from build123d import *

# Parameters (mm, degrees)
F0_R          = 3
F0_R_2        = 2.5
F1_DEPTH      = 800
F2_R          = 2
F3_R          = 7
F6_DEPTH      = 30
F6_DEPTH_BACK = 30


# Not quite as in the source:
# - a feature names something its author has since deleted; it is built from what else it names


with BuildPart() as f1:
    # F0 (on Top) → F1 (new body)
    with BuildSketch(Plane.XY):
        with BuildLine():
            Line((18.15, -30), (30, -30))
            Line((30, -30), (30, -18.15))
            Line((30, -18.15), (27.5, -18.15))
            Line((27.5, -18.15), (27.5, -20.15))
            Line((27.5, -20.15), (21.5477069044, -20.15))
            ThreePointArc((21.5477069044, -20.15), (19.5, -15), (21.5477069044, -9.85))
            Line((21.5477069044, -9.85), (27.5, -9.85))
            Line((27.5, -9.85), (27.5, -11.85))
            Line((27.5, -11.85), (30, -11.85))
            Line((30, -11.85), (30, 11.85))
            Line((30, 11.85), (27.5, 11.85))
            Line((27.5, 11.85), (27.5, 9.85))
            Line((27.5, 9.85), (21.5477069044, 9.85))
            ThreePointArc((21.5477069044, 9.85), (19.5, 15), (21.5477069044, 20.15))
            Line((21.5477069044, 20.15), (27.5, 20.15))
            Line((27.5, 20.15), (27.5, 18.15))
            Line((27.5, 18.15), (30, 18.15))
            Line((30, 18.15), (30, 30))
            Line((30, 30), (18.15, 30))
            Line((18.15, 30), (18.15, 27.5))
            Line((18.15, 27.5), (20.15, 27.5))
            Line((20.15, 27.5), (20.15, 21.5477069044))
            ThreePointArc((20.15, 21.5477069044), (15, 19.5), (9.85, 21.5477069044))
            Line((9.85, 21.5477069044), (9.85, 27.5))
            Line((9.85, 27.5), (11.85, 27.5))
            Line((11.85, 27.5), (11.85, 30))
            Line((11.85, 30), (-11.85, 30))
            Line((-11.85, 30), (-11.85, 27.5))
            Line((-11.85, 27.5), (-9.85, 27.5))
            Line((-9.85, 27.5), (-9.85, 21.5477069044))
            ThreePointArc((-9.85, 21.5477069044), (-15, 19.5), (-20.15, 21.5477069044))
            Line((-20.15, 21.5477069044), (-20.15, 27.5))
            Line((-20.15, 27.5), (-18.15, 27.5))
            Line((-18.15, 27.5), (-18.15, 30))
            Line((-18.15, 30), (-30, 30))
            Line((-30, 30), (-30, 18.15))
            Line((-30, 18.15), (-27.5, 18.15))
            Line((-27.5, 18.15), (-27.5, 20.15))
            Line((-27.5, 20.15), (-21.5477069044, 20.15))
            ThreePointArc((-21.5477069044, 20.15), (-19.5, 15), (-21.5477069044, 9.85))
            Line((-21.5477069044, 9.85), (-27.5, 9.85))
            Line((-27.5, 9.85), (-27.5, 11.85))
            Line((-27.5, 11.85), (-30, 11.85))
            Line((-30, 11.85), (-30, -11.85))
            Line((-30, -11.85), (-27.5, -11.85))
            Line((-27.5, -11.85), (-27.5, -9.85))
            Line((-27.5, -9.85), (-21.5477069044, -9.85))
            ThreePointArc((-21.5477069044, -9.85), (-19.5, -15), (-21.5477069044, -20.15))
            Line((-21.5477069044, -20.15), (-27.5, -20.15))
            Line((-27.5, -20.15), (-27.5, -18.15))
            Line((-27.5, -18.15), (-30, -18.15))
            Line((-30, -18.15), (-30, -30))
            Line((-30, -30), (-18.15, -30))
            Line((-18.15, -30), (-18.15, -27.5))
            Line((-18.15, -27.5), (-20.15, -27.5))
            Line((-20.15, -27.5), (-20.15, -21.5477069044))
            ThreePointArc((-20.15, -21.5477069044), (-15, -19.5), (-9.85, -21.5477069044))
            Line((-9.85, -21.5477069044), (-9.85, -27.5))
            Line((-9.85, -27.5), (-11.85, -27.5))
            Line((-11.85, -27.5), (-11.85, -30))
            Line((-11.85, -30), (11.85, -30))
            Line((11.85, -30), (11.85, -27.5))
            Line((11.85, -27.5), (9.85, -27.5))
            Line((9.85, -27.5), (9.85, -21.5477069044))
            ThreePointArc((9.85, -21.5477069044), (15, -19.5), (20.15, -21.5477069044))
            Line((20.15, -21.5477069044), (20.15, -27.5))
            Line((20.15, -27.5), (18.15, -27.5))
            Line((18.15, -27.5), (18.15, -30))
        make_face()
        with Locations((-25, -25)):
            Circle(F0_R, mode=Mode.SUBTRACT)
        with Locations((-15, -15)):
            Circle(F0_R_2, mode=Mode.SUBTRACT)
        with Locations((25, -25)):
            Circle(F0_R, mode=Mode.SUBTRACT)
        with Locations((15, -15)):
            Circle(F0_R_2, mode=Mode.SUBTRACT)
        with Locations((-25, 25)):
            Circle(F0_R, mode=Mode.SUBTRACT)
        with Locations((-15, 15)):
            Circle(F0_R_2, mode=Mode.SUBTRACT)
        Polygon((-7, 22), (-7, 27.5), (0, 27.5), (7, 27.5), (7, 22), (10, 16), (10, 10), (16, 10), (22, 7), (27.5, 7), (27.5, 0), (27.5, -7), (22, -7), (16, -10), (10, -10), (10, -16), (7, -22), (7, -27.5), (0, -27.5), (-7, -27.5), (-7, -22), (-10, -16), (-10, -10), (-16, -10), (-22, -7), (-27.5, -7), (-27.5, 0), (-27.5, 7), (-22, 7), (-16, 10), (-10, 10), (-10, 16), align=None, mode=Mode.SUBTRACT)
        with Locations((15, 15)):
            Circle(F0_R_2, mode=Mode.SUBTRACT)
        with Locations((25, 25)):
            Circle(F0_R, mode=Mode.SUBTRACT)
    extrude(amount=F1_DEPTH)

    # F2
    f2_edges = [f1.edges().sort_by_distance(p)[0] for p in [
        (-7, 27.5, 400),
        (7, 27.5, 400),
    ]]
    fillet(f2_edges, radius=F2_R)

    # F3
    f3_edges = [f1.edges().sort_by_distance(p)[0] for p in [
        (-10, 16, 400),
        (10, 16, 400),
    ]]
    fillet(f3_edges, radius=F3_R)

    # F5 (on Front) → F6 (cut, two sides)
    with BuildSketch(Plane.XZ) as f6_sk:
        Polygon((92.6955789172, 775.5943319306), (113.9419287111, 882.406945313), (-8.7536502061, 906.8126133825), (-30, 800), align=None)
    extrude(amount=F6_DEPTH, mode=Mode.SUBTRACT)
    extrude(f6_sk.sketch, amount=-F6_DEPTH_BACK, mode=Mode.SUBTRACT)


solid = f1.part
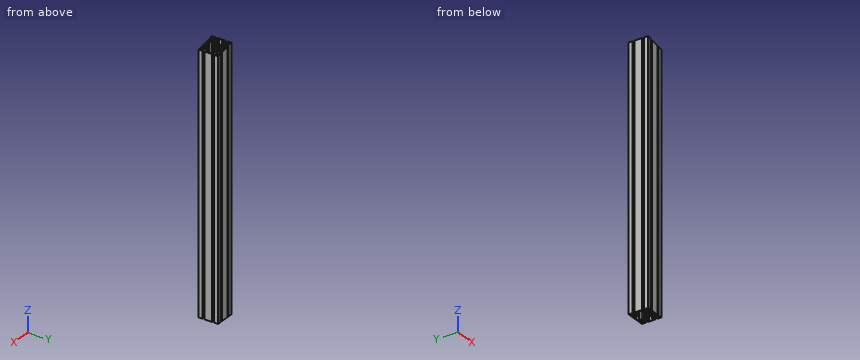
Work out the finished part from the listing and answer in its coordinate system (mm). Coordinates: 2 decimals unless noted, no trailing zeros. Use one line per item in the form item = value. Start each with the question number.
1. The part is cut by section A-A (z = 724.5). Give the number of separate pieces and of enclosed holes in the cut face, plus the area to 3 significant figures.
2. Each of these flat-tipped pins is pushed along its axis until it touches: P1, Ø1, axis at x = 12.5, z = 330.5, coming from the -Y side; P2, Ø7, axis at x = -25, y = -25, coming from the -Z side. Where does it stop, or does it pass through?
3. Straight lines are drawn through the part: probe 1 along Y at (x, z) = (-25, 500); probe 2 along Y at (x, z) = (-15, 253). For each, find the intervals that lie inside material, in ascending order. Write a range as from..to.
Evaluation:
q1.separate_pieces = 1
q1.enclosed_holes = 9
q1.area = 1,080 mm^2
q2.P1 = -20.13
q2.P2 = 0
q3.probe_1 = -30..-28, -22..-20.15, -9.85..-7, 7..9.85, 20.15..22, 28..30
q3.probe_2 = -19.5..-17.5, -12.5..-10, 10..12.5, 17.5..19.5
